Part model, mm, in its own coordinate system. A direction names the side the tool comes from. Coordinates: 2 decimals unless noted, no trailing zeros. Loops run counter-clockwise (first coordinate to the right, second up) from the corner with the lowest first, then second, coordinate; pieces in that order, holes last. Notation, with made-up numbers: M -34,-13.5 L -15,-13.5 A24 cw -15,-3.5 Z; hole C 3,-33.75 d10. An arc over 180 degrees is marked long. Use a Markdown table: item, result. Add a question column.
1) Pin check, flat tips, straight feed: pin 1 Ø1.5 at (x, z) = (0.5, 8) entering from +Y; pin 2 Ø3 at (x, y) = (-1, 2.5) entering from +Z; pin 3 Ø2 at (x, y) = (-0.5, 24) entering from -Z. Stop position of each tip, or through.
2) Tool access for faces 5 (the cylindrical face through (-0.55, 7.85, 12.77)), 6 (the flat face through (1, 24, 5.5)), 7 (the cylindrical face through (-0.454, 9.641, 29.797)): list every direction of +Z, -Z, +X, -X, +Y, -Y with a clear straight run to the whole face (end or side of a thin tool).
3) Pull direction Y, two halves, no side cores. Call faces 1 (the cylindrical face through (0.896, 27.045, 18.072)), 2 (the cylindrical face through (0.25, 22.41, 18.07)), 3 (the flat face through (-1, -4.5, 25)), 4 (the flat face through (-3.75, -2, 15)): released by +Y, released by -Y, zero draft, split by the parting line, or undercut.
4) Band-saw the part on B-B (x = -0.25). List the corners of the cut face in (y, z), plus the area to 3 significant figures.
5) Band-saw the part on D-D (z = 13.5). List the corners of the cut face in (x, y).
6) Band-saw the part on A-A (y = -12.5). List the corners of the cut face in (x, z).
7) Band-saw the part on C-C (z = 10). List the corners of the cut face in (x, y), plus the area to 3 significant figures.
8) Wall check: probe 1 along Y at (x, z) = (-0.5, 10); probe 2 along Y at (x, z) = (-1, 10); probe 3 along Y at (x, z) = (1.75, 10.5). Give the ranges that are in metal, low to high. Write a range as from..to.
from build123d import *

# Parameters (mm, degrees)
BOSS_EXTRUDE1_DEPTH = 31
SKETCH2_W           = 5.5
SKETCH2_H           = 10.5
CUT_EXTRUDE1_DEPTH  = 7.5
SKETCH3_R           = 3
CUT_EXTRUDE2_DEPTH  = 7.5
CUT_EXTRUDE4_DEPTH  = 26.5
CUT_EXTRUDE5_REACH  = 8.5
SKETCH6_W           = 8
SKETCH6_H           = 13
FILLET1_R           = 0.5
FILLET2_R           = 4


with BuildPart() as part:
    # Sketch1 → Boss-Extrude1 (new body)
    with BuildSketch(Plane.XY):
        with BuildLine():
            Line((-3.75, 29), (-3.75, 22.5))
            Line((-3.75, 22.5), (-3.75, -22.5))
            Line((-3.75, -22.5), (2.75, -22.5))
            Line((2.75, -22.5), (2.75, 22.5))
            ThreePointArc((2.75, 22.5), (0.846194078, 27.096194078), (-3.75, 29))
        make_face()
    extrude(amount=BOSS_EXTRUDE1_DEPTH)

    # Sketch2 → Cut-Extrude1 (cut, through all)
    with BuildSketch(Plane.ZY.offset(3.75)):
        with Locations((2.75, 23.75)):
            Rectangle(SKETCH2_W, SKETCH2_H)
    extrude(amount=-CUT_EXTRUDE1_DEPTH, mode=Mode.SUBTRACT)

    # Sketch3 → Cut-Extrude2 (cut, through all)
    with BuildSketch(Plane.ZY.offset(3.75)):
        with Locations((10, 9)):
            Circle(SKETCH3_R)
        with Locations((10, -12.5)):
            Circle(SKETCH3_R)
    extrude(amount=-CUT_EXTRUDE2_DEPTH, mode=Mode.SUBTRACT)

    # Sketch4 → Cut-Extrude4 (cut, through all)
    with BuildSketch(Plane(origin=(0, 0, 5.5), x_dir=(-1, 0, 0), z_dir=(0, 0, -1))):
        with BuildLine():
            Line((3.75, 26.5), (3.75, 18.5))
            ThreePointArc((3.75, 18.5), (-0.25, 22.5), (3.75, 26.5))
        make_face()
    extrude(amount=-CUT_EXTRUDE4_DEPTH, mode=Mode.SUBTRACT)

    # Sketch6 → Cut-Extrude5 (cut, up to next)
    with BuildSketch(Plane.ZY.offset(3.75), mode=Mode.PRIVATE) as cut_extrude5_sk1:
        with Locations((27, 2)):
            Rectangle(SKETCH6_W, SKETCH6_H)
    cut_extrude5_tool1 = extrude(cut_extrude5_sk1.sketch, amount=-CUT_EXTRUDE5_REACH, mode=Mode.PRIVATE) & part.part
    add(cut_extrude5_tool1.solids().sort_by_distance((-3.75, 2, 27))[0], mode=Mode.SUBTRACT)

    # Fillet1
    fillet1_edges = [part.edges().sort_by_distance(p)[0] for p in [
        (-0.5, -4.5, 23),
        (-0.5, 8.5, 23),
    ]]
    fillet(fillet1_edges, radius=FILLET1_R)

    # Fillet2
    fillet2_edges = [part.edges().sort_by_distance(p)[0] for p in [
        (-0.5, 8.5, 31),
        (-0.5, -4.5, 31),
    ]]
    fillet(fillet2_edges, radius=FILLET2_R)


solid = part.part
Entries:
| question | item | result |
|---|---|---|
| 1 | pin 1 | y = 27.98 |
| 1 | pin 2 | z = 23 |
| 1 | pin 3 | z = 5.5 |
| 2 | face 5 | +X, -X |
| 2 | face 6 | -Z, +X, -X, +Y |
| 2 | face 7 | +Z, +X, -X |
| 3 | face 1 | released by +Y |
| 3 | face 2 | undercut |
| 3 | face 3 | undercut |
| 3 | face 4 | zero draft |
| 4 | outline | M -22.5,0 L 18.5,0 L 18.5,5.5 L 20.56,5.5 L 20.56,31 L 12.5,31 A4 ccw 8.5,27 L 8.5,23.5 A0.5 cw 8,23 L -4,23 A0.5 cw -4.5,23.5 L -4.5,27 A4 ccw -8.5,31 L -22.5,31 Z; M 24.44,5.5 L 27.98,5.5 L 27.98,31 L 24.44,31 Z; hole C -12.5,10 d6; hole C 9,10 d6 |
| 4 | area | 1,250 mm2 |
| 5 | outline | M -3.75,-22.5 L 2.75,-22.5 L 2.75,22.5 A6.5 ccw -3.75,29 L -3.75,26.5 A4 cw -3.75,18.5 Z |
| 6 | outline | M -3.75,0 L 2.75,0 L 2.75,7 L -3.75,7 Z; M -3.75,13 L 2.75,13 L 2.75,31 L -3.75,31 Z |
| 7 | outline | M -3.75,-22.5 L 2.75,-22.5 L 2.75,-15.5 L -3.75,-15.5 Z; M -3.75,-9.5 L 2.75,-9.5 L 2.75,6 L -3.75,6 Z; M -3.75,12 L 2.75,12 L 2.75,22.5 A6.5 ccw -3.75,29 L -3.75,26.5 A4 cw -3.75,18.5 Z |
| 7 | area | 223 mm2 |
| 8 | probe 1 | -22.5..-15.5, -9.5..6, 12..20.17, 24.83..28.13 |
| 8 | probe 2 | -22.5..-15.5, -9.5..6, 12..19.6, 25.4..28.39 |
| 8 | probe 3 | -22.5..-15.46, -9.54..6.04, 11.96..25.96 |
